Verification items for the finished model (mm, model axes). Coordinates: 2 decimals unless noted, no trailing zeros. Write each loop counter-clockwise with the first axis right and the second up, starting at its lowest first coordinate (ties: lowest second). Pieces come first, ordered by that corner, then holes. Notation, with made-up numbers: (61, 79.25) -> (66, 79.25) arc R21 ccw to (66, 111.25) -> close; hole circle Ø7 at (75.25, -39.5). An arc over 180 degrees is marked (long way). Answer in a Markdown table with one row per item.
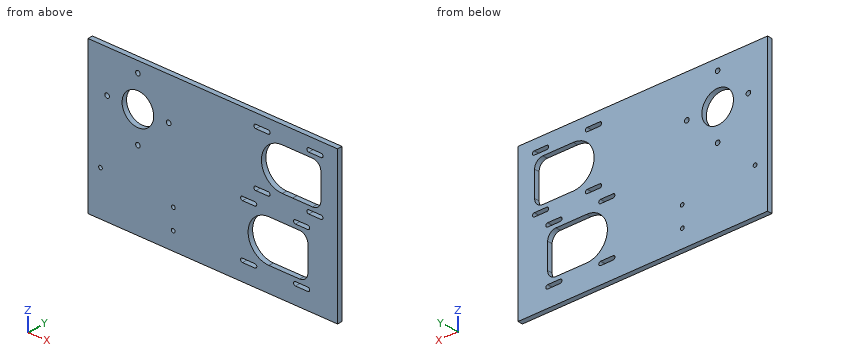
```python
from build123d import *

# Parameters (mm, degrees)
SKETCH1_W            = 290
SKETCH1_H            = 180
BOSS_EXTRUDE1_DEPTH  = 6
SKETCH2_R            = 19
CUT_EXTRUDE1_DEPTH   = 231.295462396
M4_CLEARANCE_HOLE1_D = 4.5
CUT_EXTRUDE3_DEPTH   = 10
CUT_EXTRUDE4_DEPTH   = 10
CUT_EXTRUDE5_DEPTH   = 231.295462396
FILLET1_R            = 10
SKETCH12_W           = 39.319805153
SKETCH12_H           = 50
CUT_EXTRUDE6_DEPTH   = 10
FILLET2_R            = 10
CIRPATTERN1_COUNT    = 4
SKETCH15_W           = 180
SKETCH15_H           = 6
BOSS_EXTRUDE2_DEPTH  = 10


with BuildPart() as part:
    # Sketch1 → Boss-Extrude1 (new body)
    with BuildSketch(Plane(origin=(0, 0, 0), x_dir=(1, 0, 0), z_dir=(0, 1, 0))):
        with Locations((45, 40)):
            Rectangle(SKETCH1_W, SKETCH1_H)
    extrude(amount=BOSS_EXTRUDE1_DEPTH)

    # Sketch2 → Cut-Extrude1 (cut, through all)
    with BuildSketch(Plane(origin=(0, 6, 0), x_dir=(1, 0, 0), z_dir=(0, 1, 0))):
        with Locations(Location((-50, 0, 0), (0, 0, 270))):
            Circle(SKETCH2_R)
    extrude(amount=-CUT_EXTRUDE1_DEPTH, mode=Mode.SUBTRACT)

    # M4 Clearance Hole1 (through all)
    with Locations(Plane(origin=(0, 6, 0), x_dir=(1, 0, 0), z_dir=(0, 1, 0))):
        with Locations((-95, 77), (-7.608586267, 108.807873329), (-7.334866568, 84.669705362)):
            Hole(M4_CLEARANCE_HOLE1_D / 2)

    # Sketch8 → Cut-Extrude3 (cut)
    with BuildSketch(Plane(origin=(0, 6, 0), x_dir=(1, 0, 0), z_dir=(0, 1, 0))):
        with BuildLine():
            Line((75.680194847, 110.069805153), (90.680194847, 110.069805153))
            ThreePointArc((90.680194847, 110.069805153), (92.930194847, 107.819805153), (90.680194847, 105.569805153))
            Line((90.680194847, 105.569805153), (75.680194847, 105.569805153))
            ThreePointArc((75.680194847, 105.569805153), (73.430194847, 107.819805153), (75.680194847, 110.069805153))
        make_face()
        with BuildLine():
            Line((139.319805153, 110.069805153), (154.319805153, 110.069805153))
            ThreePointArc((154.319805153, 110.069805153), (156.569805153, 107.819805153), (154.319805153, 105.569805153))
            Line((154.319805153, 105.569805153), (139.319805153, 105.569805153))
            ThreePointArc((139.319805153, 105.569805153), (137.069805153, 107.819805153), (139.319805153, 110.069805153))
        make_face()
        with BuildLine():
            Line((75.680194847, 46.430194847), (90.680194847, 46.430194847))
            ThreePointArc((90.680194847, 46.430194847), (92.930194847, 44.180194847), (90.680194847, 41.930194847))
            Line((90.680194847, 41.930194847), (75.680194847, 41.930194847))
            ThreePointArc((75.680194847, 41.930194847), (73.430194847, 44.180194847), (75.680194847, 46.430194847))
        make_face()
        with BuildLine():
            Line((139.319805153, 46.430194847), (154.319805153, 46.430194847))
            ThreePointArc((154.319805153, 46.430194847), (156.569805153, 44.180194847), (154.319805153, 41.930194847))
            Line((154.319805153, 41.930194847), (139.319805153, 41.930194847))
            ThreePointArc((139.319805153, 41.930194847), (137.069805153, 44.180194847), (139.319805153, 46.430194847))
        make_face()
        with BuildLine():
            Line((107.5, 101), (122.5, 101))
            ThreePointArc((122.5, 101), (147.5, 76), (122.5, 51))
            Line((122.5, 51), (107.5, 51))
            ThreePointArc((107.5, 51), (82.5, 76), (107.5, 101))
        make_face()
    extrude(amount=-CUT_EXTRUDE3_DEPTH, mode=Mode.SUBTRACT)

    # Sketch9 → Cut-Extrude4 (cut)
    with BuildSketch(Plane(origin=(0, 6, 0), x_dir=(1, 0, 0), z_dir=(0, 1, 0))):
        with BuildLine():
            Line((91.680194847, 30.069805153), (106.680194847, 30.069805153))
            ThreePointArc((106.680194847, 30.069805153), (108.930194847, 27.819805153), (106.680194847, 25.569805153))
            Line((106.680194847, 25.569805153), (91.680194847, 25.569805153))
            ThreePointArc((91.680194847, 25.569805153), (89.430194847, 27.819805153), (91.680194847, 30.069805153))
        make_face()
        with BuildLine():
            Line((155.319805153, 30.069805153), (170.319805153, 30.069805153))
            ThreePointArc((170.319805153, 30.069805153), (172.569805153, 27.819805153), (170.319805153, 25.569805153))
            Line((170.319805153, 25.569805153), (155.319805153, 25.569805153))
            ThreePointArc((155.319805153, 25.569805153), (153.069805153, 27.819805153), (155.319805153, 30.069805153))
        make_face()
        with BuildLine():
            Line((91.680194847, -33.569805153), (106.680194847, -33.569805153))
            ThreePointArc((106.680194847, -33.569805153), (108.930194847, -35.819805153), (106.680194847, -38.069805153))
            Line((106.680194847, -38.069805153), (91.680194847, -38.069805153))
            ThreePointArc((91.680194847, -38.069805153), (89.430194847, -35.819805153), (91.680194847, -33.569805153))
        make_face()
        with BuildLine():
            Line((155.319805153, -33.569805153), (170.319805153, -33.569805153))
            ThreePointArc((170.319805153, -33.569805153), (172.569805153, -35.819805153), (170.319805153, -38.069805153))
            Line((170.319805153, -38.069805153), (155.319805153, -38.069805153))
            ThreePointArc((155.319805153, -38.069805153), (153.069805153, -35.819805153), (155.319805153, -33.569805153))
        make_face()
        with BuildLine():
            Line((123.5, 21), (138.5, 21))
            ThreePointArc((138.5, 21), (163.5, -4), (138.5, -29))
            Line((138.5, -29), (123.5, -29))
            ThreePointArc((123.5, -29), (98.5, -4), (123.5, 21))
        make_face()
    extrude(amount=-CUT_EXTRUDE4_DEPTH, mode=Mode.SUBTRACT)

    # Sketch10 → Cut-Extrude5 (cut, through all)
    with BuildSketch(Plane(origin=(0, 6, 0), x_dir=(1, 0, 0), z_dir=(0, 1, 0))):
        with BuildLine():
            Line((123.5, 21), (136, 21.004881403))
            Line((136, 21.004881403), (170, 21.004881403))
            Line((170, 21.004881403), (170, -29))
            Line((170, -29), (136, -29))
            Line((136, -29), (123.5, -29))
            ThreePointArc((123.5, -29), (98.5, -4), (123.5, 21))
        make_face()
    extrude(amount=-CUT_EXTRUDE5_DEPTH, mode=Mode.SUBTRACT)

    # Fillet1
    fillet1_edges = [part.edges().sort_by_distance(p)[0] for p in [
        (170, 3, 29),
        (170, 3, -21.004881403),
    ]]
    fillet(fillet1_edges, radius=FILLET1_R)

    # Sketch12 → Cut-Extrude6 (cut)
    with BuildSketch(Plane(origin=(0, 6, 0), x_dir=(1, 0, 0), z_dir=(0, 1, 0))):
        with Locations((134.659902577, 76)):
            Rectangle(SKETCH12_W, SKETCH12_H)
    extrude(amount=-CUT_EXTRUDE6_DEPTH, mode=Mode.SUBTRACT)

    # Fillet2
    fillet2_edges = [part.edges().sort_by_distance(p)[0] for p in [
        (154.319805153, 3, -51),
        (154.319805153, 3, -101),
    ]]
    fillet(fillet2_edges, radius=FILLET2_R)

    # Sketch14 → M5 Clearance Hole2 (revolve, cut)
    with BuildSketch(Plane(origin=(-13, 6, 0), x_dir=(0, 0, 1), z_dir=(1, 0, 0))):
        Polygon((0, 0), (0, 21.652366702), (2.75, 20), (2.75, 0), align=None)
    m5_clearance_hole2 = revolve(axis=Axis((-13, 12.35, 0), (0, -1, 0)), mode=Mode.SUBTRACT)

    # CirPattern1: M5 Clearance Hole2 ×4 about axis
    cirpattern1_axis = Axis((-50, 0, 0), (0, 1, 0))
    for i in range(1, CIRPATTERN1_COUNT):
        add(m5_clearance_hole2.rotate(cirpattern1_axis, i * 360 / CIRPATTERN1_COUNT), mode=Mode.SUBTRACT)

    # Sketch15 → Boss-Extrude2 (add)
    with BuildSketch(Plane.ZY.offset(100)):
        with Locations((-40, 3)):
            Rectangle(SKETCH15_W, SKETCH15_H)
    extrude(amount=BOSS_EXTRUDE2_DEPTH)


solid = part.part
```
1. Sectioned sample at B-B, the plane z = -56.5. Record the cut outline in (x, y).
Findings below:
| item | result |
|---|---|
| outline | (-110, 0) -> (91.86, 0) -> (91.86, 6) -> (-110, 6) -> close; (153.25, 0) -> (190, 0) -> (190, 6) -> (153.25, 6) -> close |
2. Material ranges on probe 1 along X at (y, z) = (3.75, -77); probe 2 along Z at (x, y) = (164, 0.55); probe 3 along X at (y, z) = (3, -37), recorded low to high. Write a range as from..to.
Findings below:
| item | result |
|---|---|
| probe 1 | x = -110..-97.25, -92.75..82.52, 154.32..190 |
| probe 2 | z = -130..-30.07, -25.57..-20.17, 28.17..33.57, 38.07..50 |
| probe 3 | x = -110..-52.75, -47.25..190 |
3. Sectioned sample at A-A, the plane z = -6. Record the cut outline in (x, y).
Findings below:
| item | result |
|---|---|
| outline | (-110, 0) -> (-68.03, 0) -> (-68.03, 6) -> (-110, 6) -> close; (-31.97, 0) -> (100.59, 0) -> (100.59, 6) -> (-31.97, 6) -> close; (170, 0) -> (190, 0) -> (190, 6) -> (170, 6) -> close |
4. Go/stop test with a flat-tipped pin: pin 1 (3.5 mm diameter, centred on x = -50, z = -37, fed in from -Y). Record where the tip stops, or that it passes through.
Findings below:
| item | result |
|---|---|
| pin 1 | passes through |
5. Sectioned sample at C-C, the plane y = 2.45. Count the separate pieces of the cut face and the enclosed holes in it, and give its area (3 significant figures).
Findings below:
| item | result |
|---|---|
| separate pieces | 1 |
| enclosed holes | 18 |
| area | 45,500 mm² |
